from build123d import *

# Parameters (mm, degrees)
F0_W           = 70
F0_H           = 50
F1_DEPTH       = 2
F3_W           = 1.5
F3_H           = 12.5
F4_DEPTH       = 4.5
F5_D           = 3
F5_DEPTH       = 10
F5_TIP         = 0.9012909285
F5_ON_F3_D     = 3
F5_ON_F3_DEPTH = 10
F5_ON_F3_TIP   = 0.9012909285
F3_W_2         = 10
F3_H_2         = 5
F3_W_3         = 2
F3_H_3         = 8
F3_H_4         = 20
F6_DEPTH       = 3


with BuildPart() as f1:
    # F0 (on Top) → F1 (new body)
    with BuildSketch(Plane.XY):
        Rectangle(F0_W, F0_H)
    extrude(amount=F1_DEPTH)

    # F3 (on face) → F4 (join)
    with BuildSketch(Plane.XY.offset(2)):
        with Locations((-29.875, 6.25)):
            Rectangle(F3_W, F3_H)
        with Locations((-29.875, -6.25)):
            Rectangle(F3_W, F3_H)
        with Locations((-7.375, 6.25)):
            Rectangle(F3_W, F3_H)
        with Locations((-7.375, -6.25)):
            Rectangle(F3_W, F3_H)
    extrude(amount=F4_DEPTH)

    # F5
    with Locations(Plane.XY.offset(2)):
        with Locations((-0.5, 15.5), (30, 15.5), (30, -15), (-0.5, -15)):
            Hole(F5_D / 2, depth=F5_DEPTH)
            with Locations((0, 0, -(F5_DEPTH + F5_TIP / 2))):  # 118° drill point
                Cone(0, F5_D / 2, F5_TIP, mode=Mode.SUBTRACT)

    # F5 on F3
    with Locations(Plane.XY.offset(2)):
        with Locations((-5.125, 0), (-32.125, 0)):
            Hole(F5_ON_F3_D / 2, depth=F5_ON_F3_DEPTH)
            with Locations((0, 0, -(F5_ON_F3_DEPTH + F5_ON_F3_TIP / 2))):  # 118° drill point
                Cone(0, F5_ON_F3_D / 2, F5_ON_F3_TIP, mode=Mode.SUBTRACT)

    # F3 (on face) → F6 (join)
    with BuildSketch(Plane.XY.offset(2)):
        with Locations((-18.625, 10)):
            Rectangle(F3_W_2, F3_H_2)
        with Locations((-18.625, -10)):
            Rectangle(F3_W_2, F3_H_2)
        with Locations((26.5, -15)):
            Rectangle(F3_W_3, F3_H_2)
        with Locations((30, 8)):
            Rectangle(F3_W_3, F3_H_3)
        with Locations((-0.5, 0.25)):
            Rectangle(F3_W_3, F3_H_4)
    extrude(amount=F6_DEPTH)


solid = f1.part
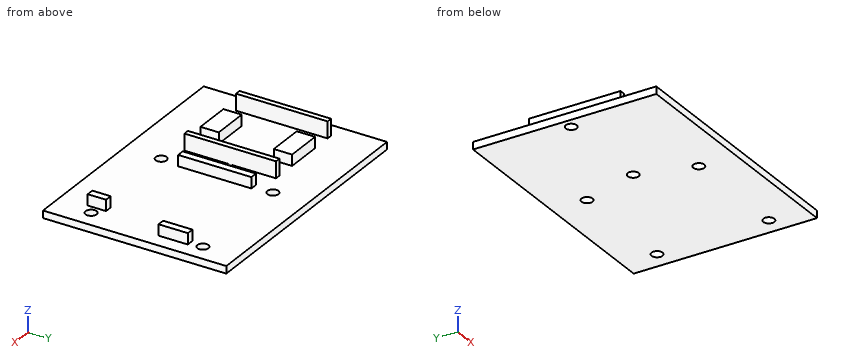
For this review, take the finished solid that the model builds, in its own axes (mm). Round coordinates to 2 decimals unless told otherwise and drop trailing zeros. Write each loop counter-clockwise with the first axis right and the second up, starting at its lowest first coordinate (ties: lowest second). Pieces come first, ordered by that corner, then holes. Notation, with made-up numbers: M -33.75,81 L -5.75,81 A21 cw -5.75,90 Z; hole C 53.5,21.25 d2. An arc over 180 degrees is marked long. Write item = value, one per line. Start each with the question number.
(1) Clearance check with flat-ended pins moving along their axes: pin 1 Ø2 at (y, z) = (2, 4.5) entering from -X (3 decimals); pin 2 Ø0.9 at (y, z) = (-16, 4) entering from -X; pin 3 Ø2.5 at (y, z) = (-9, 3.5) entering from +X; pin 4 Ø2.5 at (x, y) = (30, 15.5) entering from +Z. State where each tip first meets the part, or that it passes through.
(2) We need section B-B (y = -15). Give the boundary of the cut face in (x, z).
(3) For line 1 along Y through (x, z) = (30, 1.25); line 2 along X through (y, z) = (-1.5, 3.5) (3 decimals); line 3 along Y through (x, z) = (-20.5, 3.25), list the stretches that pass through material, from the lowest coordinate up.
(4) We need section C-C (x = -0.5). Give the boundary of the cut face in (y, z).
(5) We need section A-A (z = 3.5). Give the boundary of the cut face in (x, y) (3 decimals), then the cut area to 3 significant figures.
(6) We need section D-D (y = -4). Give the boundary of the cut face in (x, z) (3 decimals).
Results found:
q1.pin_1 = -30.625
q1.pin_2 = 25.5
q1.pin_3 = 0.5
q1.pin_4 = through
q2.outline = M -35,0 L -2,0 L -2,2 L -35,2 Z; M 1,0 L 28.5,0 L 28.5,2 L 27.5,2 L 27.5,5 L 25.5,5 L 25.5,2 L 1,2 Z; M 31.5,0 L 35,0 L 35,2 L 31.5,2 Z
q3.line_1 = -25 to -16.5, -13.5 to 14, 17 to 25
q3.line_2 = -30.625 to -29.125, -8.125 to -6.625, -1.5 to 0.5
q3.line_3 = -12.5 to -7.5, 7.5 to 12.5
q4.outline = M -25,0 L -16.5,0 L -16.5,2 L -25,2 Z; M -13.5,0 L 14,0 L 14,2 L 10.25,2 L 10.25,5 L -9.75,5 L -9.75,2 L -13.5,2 Z; M 17,0 L 25,0 L 25,2 L 17,2 Z
q5.outline = M -30.625,-12.5 L -29.125,-12.5 L -29.125,12.5 L -30.625,12.5 Z; M -23.625,-12.5 L -13.625,-12.5 L -13.625,-7.5 L -23.625,-7.5 Z; M -23.625,7.5 L -13.625,7.5 L -13.625,12.5 L -23.625,12.5 Z; M -8.125,-12.5 L -6.625,-12.5 L -6.625,12.5 L -8.125,12.5 Z; M -1.5,-9.75 L 0.5,-9.75 L 0.5,10.25 L -1.5,10.25 Z; M 25.5,-17.5 L 27.5,-17.5 L 27.5,-12.5 L 25.5,-12.5 Z; M 29,4 L 31,4 L 31,12 L 29,12 Z
q5.area = 241 mm²
q6.outline = M -35,0 L 35,0 L 35,2 L 0.5,2 L 0.5,5 L -1.5,5 L -1.5,2 L -6.625,2 L -6.625,6.5 L -8.125,6.5 L -8.125,2 L -29.125,2 L -29.125,6.5 L -30.625,6.5 L -30.625,2 L -35,2 Z
